```python
from build123d import *

# Parameters (mm, degrees)
BASE_FLANGE1_DEPTH = 3
CUT_EXTRUDE1_DEPTH = 10


# Sheet-metal steps are written as plain solids
with BuildPart() as part:
    # Sketch1 → Base-Flange1 (new body)
    with BuildSketch(Plane.XY):
        with BuildLine():
            Line((5, 10), (41, 10))
            ThreePointArc((41, 10), (46, 0), (41, -10))
            Line((41, -10), (5, -10))
            ThreePointArc((5, -10), (0, 0), (5, 10))
        make_face()
    extrude(amount=-BASE_FLANGE1_DEPTH)

    # Sketch4 → Cut-Extrude1 (cut)
    with BuildSketch(Plane.XY):
        with BuildLine():
            Line((5.5, 3), (5.5, -3))
            ThreePointArc((5.5, -3), (9.75, -5), (14, -3))
            Line((14, -3), (14, 3))
            ThreePointArc((14, 3), (9.75, 5), (5.5, 3))
        make_face()
        with BuildLine():
            Line((39, 4.25), (33, 4.25))
            ThreePointArc((33, 4.25), (31, 0), (33, -4.25))
            Line((33, -4.25), (39, -4.25))
            ThreePointArc((39, -4.25), (41, 0), (39, 4.25))
        make_face()
    extrude(amount=-CUT_EXTRUDE1_DEPTH, mode=Mode.SUBTRACT)


solid = part.part
```
Model file for the job. Use its own axes, mm. A direction names the side the tool comes from. Round coordinates to 2 decimals unless told otherwise and drop trailing zeros. Write each loop counter-clockwise with the first axis right and the second up, starting at its lowest first coordinate (ties: lowest second). Pieces come first, ordered by that corner, then holes. Notation, with made-up numbers: (13, -9.75) - (46, -9.75) arc R9 ccw to (46, 2.25) - close; hole circle Ø1 at (-35.75, -28.5). An arc over 180 degrees is marked (long way). Use CSV: the item, a comma, the result in double quotes. Start each with the question number.
Item 1: Band-saw the part on C-C (y = -3.5). Write the cut outline in (x, z), and give its area (3 significant figures).
Item 2: Tool access for faces 1 (the face through (14, 0, -1)), 2 (the face through (23, 10, -1)): list every direction of +Z, -Z, +X, -X, +Y, -Y with a clear straight run to the whole face (end or side of a thin tool).
Item 3: Two-plate mould, pull along Y, no slides. Class faces 3 (the face through (46, 0, -1)), 4 (the face through (23, 0, 0)), 5 (the face through (9.7, -5, -1.5)): released by +Y, released by -Y, zero draft, split by the parting line, or undercut.
Item 4: Pin check, flat tips, straight feed: P1, Ø1, axis at y = -3.5, z = -2, coming from the +X side; P2, Ø1, axis at y = 8, z = -2.5, coming from the -X side; P3, Ø1.5, axis at y = -6, z = -1, coming from the +X side. Stop position of each tip, or through.
Item 5: Band-saw the part on A-A (x = 37). Write the cut outline in (y, z), and give its area (3 significant figures).
Item 6: Band-saw the part on B-B (z = -2.05). Write the cut outline in (x, y).
Item 7: Drill centre lines: L1, parallel to X at y = -2.25, z = -0.3; L2, parallel to X at y = 0.75, z = -1.1; L3, parallel to Y at x = 13.5, z = -1.75. Where is each one in solid material? Low to high. Write a range as [from, to].
Item 8: Band-saw the part on D-D (x = 13). Write the cut outline in (y, z), and give its area (3 significant figures).
Checked values:
1,outline,"(0.5, -3) - (5.97, -3) - (5.97, 0) - (0.5, 0) - close; (13.53, -3) - (32.25, -3) - (32.25, 0) - (13.53, 0) - close; (39.75, -3) - (45.5, -3) - (45.5, 0) - (39.75, 0) - close"
1,area,"89.8 mm²"
2,face 1,"+Z, -Z"
2,face 2,"+Z, -Z, +X, -X, +Y"
3,face 3,"split by the parting line"
3,face 4,"zero draft"
3,face 5,"undercut"
4,P1,"stops at x = 45.63"
4,P2,"stops at x = 2.5"
4,P3,"stops at x = 44.84"
5,outline,"(-10, -3) - (-4.25, -3) - (-4.25, 0) - (-10, 0) - close; (4.25, -3) - (10, -3) - (10, 0) - (4.25, 0) - close"
5,area,"34.5 mm²"
6,outline,"(5, -10) - (41, -10) arc R12.5 ccw to (41, 10) - (5, 10) arc R12.5 ccw to start; hole (5.5, -3) arc R5.52 ccw to (14, -3) - (14, 3) arc R5.52 ccw to (5.5, 3) - close; hole (33, -4.25) - (39, -4.25) arc R5.52 ccw to (39, 4.25) - (33, 4.25) arc R5.52 ccw to start"
7,L1,"x = [0.2, 5.5], [14, 31.48], [40.52, 45.8]"
7,L2,"x = [0.02, 5.5], [14, 31.05], [40.95, 45.98]"
7,L3,"y = [-10, -3.53], [3.53, 10]"
8,outline,"(-10, -3) - (-3.94, -3) - (-3.94, 0) - (-10, 0) - close; (3.94, -3) - (10, -3) - (10, 0) - (3.94, 0) - close"
8,area,"36.4 mm²"
